For this review, take the finished solid that the model builds, in its own axes (mm). Round coordinates to 2 decimals unless told otherwise and drop trailing zeros. Write each loop counter-clockwise with the first axis right and the second up, starting at its lowest first coordinate (ties: lowest second). Pieces come first, ordered by that corner, then holes. Notation, with made-up numbers: M 22.5,62.5 L 43.5,62.5 A16 cw 43.5,84.5 Z; hole C 35.25,-37 d3. An arc over 180 degrees is marked long. Write each question's results on one line, items separated by ' | '. Start each with the question number.
```python
from build123d import *

# Parameters (mm, degrees)
F0_W     = 101.6
F0_H     = 38.1
F1_DEPTH = 3.175
F3_DEPTH = 254
F2_R     = 3.81
F2_R_2   = 3.175
F4_DEPTH = 101.6
F5_DEPTH = 19.05
F6_START = -39.37
F6_DEPTH = 22.86
F7_START = -82.55
F7_DEPTH = 19.05


with BuildPart() as f1:
    # F0 (on Top) → F1 (new body)
    with BuildSketch(Plane.XY):
        with Locations((-50.8, -19.05)):
            Rectangle(F0_W, F0_H)
    extrude(amount=F1_DEPTH)

    # F2 (on face) → F3 (cut)
    with BuildSketch(Plane(origin=(-101.6, 0, 0), x_dir=(0, -1, 0), z_dir=(-1, 0, 0))):
        with BuildLine():
            ThreePointArc((3.7567106623, 3.175), (3.7966542918, 3.4913839483), (3.81, 3.81))
            ThreePointArc((3.81, 3.81), (-2.6940768363, 6.5040768363), (0, 0))
            Line((0, 0), (0, 0.635))
            ThreePointArc((0, 0.635), (-2.2450640303, 6.0550640303), (3.175, 3.81))
            ThreePointArc((3.175, 3.81), (3.1589222858, 3.4908840456), (3.1108519733, 3.175))
            Line((3.1108519733, 3.175), (3.7567106623, 3.175))
        make_face()
        with BuildLine():
            Line((0, 0.635), (0, 0))
            ThreePointArc((0, 0), (2.4593444248, 0.9000644337), (3.7567106623, 3.175))
            Line((3.7567106623, 3.175), (3.1108519733, 3.175))
            ThreePointArc((3.1108519733, 3.175), (2.0080463142, 1.3506555752), (0, 0.635))
        make_face()
        with BuildLine():
            Line((0, 3.175), (0, 0.635))
            ThreePointArc((0, 0.635), (2.0080463142, 1.3506555752), (3.1108519733, 3.175))
            Line((3.1108519733, 3.175), (0, 3.175))
        make_face()
    extrude(amount=-F3_DEPTH, mode=Mode.SUBTRACT)

    # F2 (on face) → F4 (join, through all)
    with BuildSketch(Plane(origin=(-101.6, 0, 0), x_dir=(0, -1, 0), z_dir=(-1, 0, 0))):
        with Locations((0, 3.81)):
            Circle(F2_R)
        with Locations((0, 3.81)):
            Circle(F2_R_2, mode=Mode.SUBTRACT)
    extrude(amount=-F4_DEPTH)

    # F2 (on face) → F5 (cut)
    with BuildSketch(Plane(origin=(-101.6, 0, 0), x_dir=(0, -1, 0), z_dir=(-1, 0, 0))):
        with Locations((0, 3.81)):
            Circle(F2_R)
        with Locations((0, 3.81)):
            Circle(F2_R_2, mode=Mode.SUBTRACT)
    extrude(amount=-F5_DEPTH, mode=Mode.SUBTRACT)

    # F2 (on face) → F6 (cut)
    with BuildSketch(Plane(origin=(-101.6, 0, 0), x_dir=(0, -1, 0), z_dir=(-1, 0, 0)).offset(F6_START)):
        with Locations((0, 3.81)):
            Circle(F2_R)
        with Locations((0, 3.81)):
            Circle(F2_R_2, mode=Mode.SUBTRACT)
    extrude(amount=-F6_DEPTH, mode=Mode.SUBTRACT)

    # F2 (on face) → F7 (cut)
    with BuildSketch(Plane(origin=(-101.6, 0, 0), x_dir=(0, -1, 0), z_dir=(-1, 0, 0)).offset(F7_START)):
        with Locations((0, 3.81)):
            Circle(F2_R)
        with Locations((0, 3.81)):
            Circle(F2_R_2, mode=Mode.SUBTRACT)
    extrude(amount=-F7_DEPTH, mode=Mode.SUBTRACT)


solid = f1.part
```
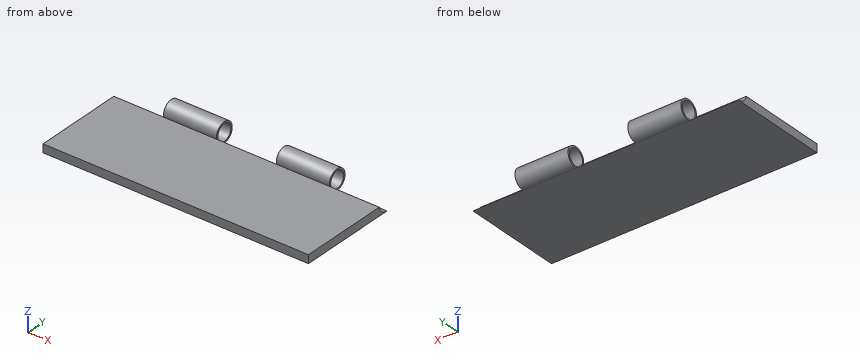
Item 1: We need section B-B on x = -15. State the section outline as (y, z) points (3 decimals), then the cut area to 3 significant figures.
Item 2: We need section C-C on y = -28. State the section outline as (x, z) points (3 decimals).
Item 3: We need section A-A on x = -80. State the section outline as (y, z) points (3 decimals), then the cut area to 3 significant figures.
Item 4: Insertion check: P1, Ø3, axis at x = -47, y = -5.5, coming from the -Z side; P2, Ø4, axis at x = -21.5, y = -13.5, coming from the +Z side (3 decimals); P3, Ø2.5, axis at y = -1.5, z = 3, coming from the +X side; P4, Ø2, axis at x = -66.5, z = 5.5, coming from the -Y side. Each pin has a flat end and moves straight along its axis. Give the tip position at first contact, or say it passes through.
Item 5: For probe 1 along Z at (x, y) = (-73.75, 0) (3 decimals); probe 2 along X at (y, z) = (-3, 2.5); probe 3 along Z at (x, y) = (-19, -26.5) (3 decimals), list the stretches that pass through material, from the lowest coordinate up.
Numbers:
1) outline: M -38.1,0 L 0,0 A3.81 cw -3.757,3.175 L -38.1,3.175 Z | area: 112 mm^2
2) outline: M -101.6,0 L 0,0 L 0,3.175 L -101.6,3.175 Z
3) outline: M -38.1,0 L 0,0 A3.81 ccw long -3.757,3.175 L -38.1,3.175 Z; hole C 0,3.81 d6.35 | area: 126 mm^2
4) P1: stops at z = 0 | P2: stops at z = 3.175 | P3: passes through | P4: stops at y = -3.75
5) probe 1: z = 0 to 0.635, 6.985 to 7.62 | probe 2: x = -82.55 to -62.23, -39.37 to -19.05 | probe 3: z = 0 to 3.175
